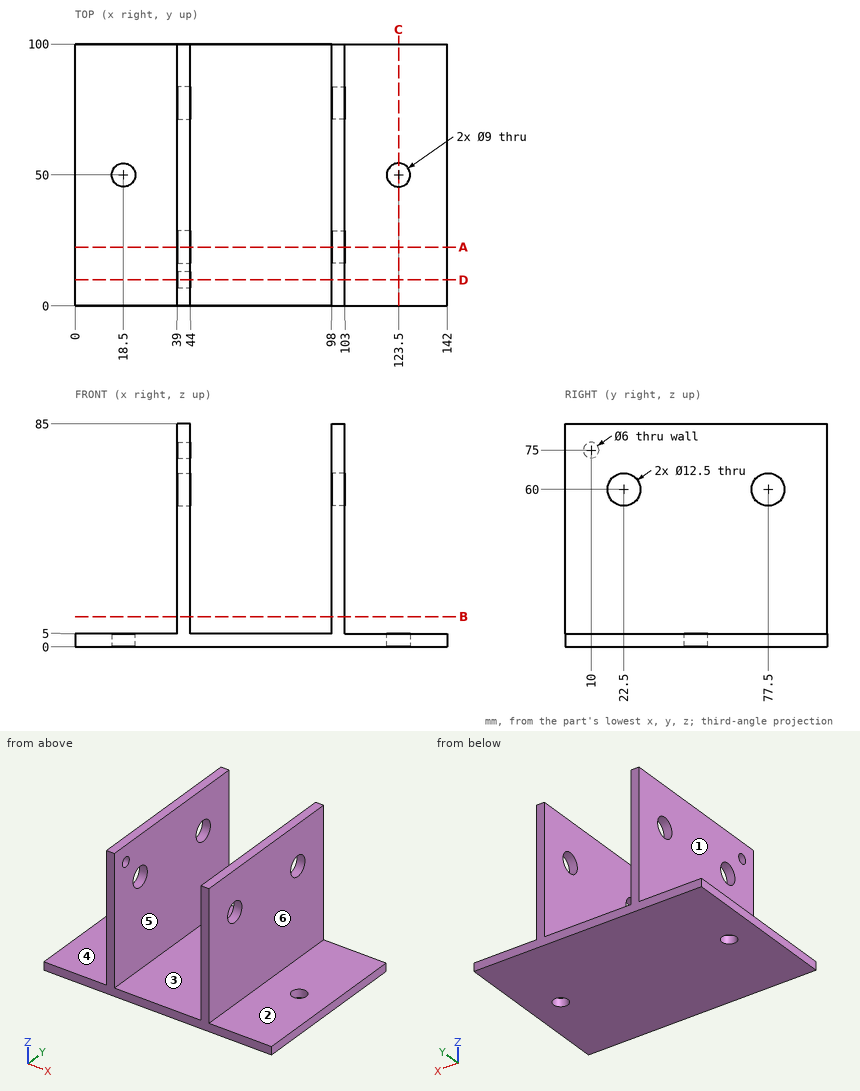
Design review of the part shown in the three views and the two pictorial views. Dimensions are in mm from the part's minimum x, y and z. A direction names the side the tool comes from. Round coordinates to 2 decimals unless told otherwise and drop trailing zeros. Write each loop counter-clockwise with the first axis right and the second up, starting at its lowest first coordinate (ties: lowest second). Pieces come first, ordered by that corner, then holes. Notation, with made-up numbers: M 30,-17.5 L 49,-17.5 A32 cw 49,19.5 Z; hole C -31.75,50 d4. An arc over 180 degrees is marked long. One line per item, written item: value. Start each with the question number.
1. Take a section at A-A on y = 22.5. State the section outline as (x, z) points, then the cut area to 4 significant figures.
2. Take a section at B-B on z = 11.5. State the section outline as (x, y) points, then the cut area to 3 significant figures.
3. Draft analysis for pull direction X (two halves, no side actions). For the marked faces 4, 5 and 6, state which applies: pulls with the +X half, pulls with the -X half, needs draft (parallel to the pull), parting line crosses it, or undercut.
4. Take a section at D-D on y = 10. State the section outline as (x, z) points, then the cut area to 3 significant figures.
5. Clearance check with flat-ended pins moving along their axes: P1, Ø4, axis at y = 33.5, z = 48, coming from the +X side; P2, Ø16, axis at y = 22.5, z = 60, coming from the -X side. State where each tip first meets the part, or that it passes through.
6. To check wall thickness, follow probe 1 along Y at (x, z) = (99, 60); probe 2 along X at (y, z) = (71, 71.5); probe 3 along Y at (x, z) = (41, 62). State the ranges of each line that lie inside material, in increasing order. Write a range as from..to.
7. For the marked faces 1, 2 and 3, list the 3-axis set-ups (+Z, -Z, +X, -X, +Y, -Y) from which the entire face can be reached by the end or side of a thin tool; tool diameter is ignored.
8. Take a section at C-C on x = 123.5. State the section outline as (y, z) points, then the cut area to 3 significant figures.
Computed:
1. outline: M 0,0 L 142,0 L 142,5 L 103,5 L 103,53.75 L 98,53.75 L 98,5 L 44,5 L 44,53.75 L 39,53.75 L 39,5 L 0,5 Z; M 39,66.25 L 44,66.25 L 44,85 L 39,85 Z; M 98,66.25 L 103,66.25 L 103,85 L 98,85 Z
1. area: 1,385 mm²
2. outline: M 39,0 L 44,0 L 44,100 L 39,100 Z; M 98,0 L 103,0 L 103,100 L 98,100 Z
2. area: 1,000 mm²
3. face 4: needs draft
3. face 5: undercut
3. face 6: pulls with the +X half
4. outline: M 0,0 L 142,0 L 142,5 L 103,5 L 103,85 L 98,85 L 98,5 L 44,5 L 44,72 L 39,72 L 39,5 L 0,5 Z; M 39,78 L 44,78 L 44,85 L 39,85 Z
4. area: 1,480 mm²
5. P1: stops at x = 103
5. P2: stops at x = 39
6. probe 1: y = 0..16.25, 28.75..71.25, 83.75..100
6. probe 2: x = 39..44, 98..103
6. probe 3: y = 0..16.58, 28.42..71.58, 83.42..100
7. face 1: +Z, -X, +Y, -Y
7. face 2: +Z, +X, +Y, -Y
7. face 3: +Z, +Y, -Y
8. outline: M 0,0 L 45.5,0 L 45.5,5 L 0,5 Z; M 54.5,0 L 100,0 L 100,5 L 54.5,5 Z
8. area: 455 mm²
